Could you check a few things on this model? Use its own coordinates, in mm. A direction names the side the tool comes from. Give positions to 0.01 mm unless a question says otherwise; leave off trailing zeros. Order: outer loops, then holes, each group sorted by start corner. A loop starts at its lowest first (then second) coordinate and runs counter-clockwise, first axis right, second up. Notation, with made-up numbers: (-24, -34.5) -> (17, -34.5) arc R23 cw to (17, -23.5) -> close; hole circle Ø9 at (87, 12). An arc over 180 degrees is marked (long way). Answer as CSV lines item,"result". Start each with the question number.
(1) Will these pins go through, and if not, where does the flat tip stop? pin 1 Ø3 at (x, z) = (7, 27) entering from +Y; pin 2 Ø8.5 at (x, y) = (1.5, 32.5) entering from +Z; pin 3 Ø6.5 at (x, y) = (0, 38) entering from +Z; pin 4 Ø8 at (x, z) = (-3.5, 29.5) entering from -Y.
(2) I want a section at D-D (z = 25.5). Please give me the cut outline in (x, y), plus the area to 3 significant figures.
(3) On a 3-axis mill with a long thin cutter (end or side, diameter ignored), from which of +Z, -Z, +X, -X, +Y, -Y can I reach the whole of each face in a straight line? I mean faces 4 (the face through (-1.2, 0.3, 13.4)), 5 (the face through (0, 2, 26)). Say none if no direction works.
(4) I want a section at C-C (x = -4.5). Please give me the cut outline in (y, z).
(5) I need wall thicknesses on L1, parallel to X at y = 0.35, z = 38; L2, parallel to Y at x = -2, z = 3.5. Which ranges of each line are inside material? Lowest first, please.
(6) We'd pull the mould along Y, two halves only. Please class faces 1 (the face through (-5.94, 0.99, 47.58)), 2 (the face through (-0.12, 0.86, 0.9)), 3 (the face through (-0.434, 36.048, 0.254)): released by +Y, released by -Y, zero draft, split by the parting line, or undercut.
(7) I want a section at A-A (y = 38). Please give me the cut outline in (x, z).
```python
from build123d import *

# Parameters (mm, degrees)
EXTRUDE_1_DEPTH      = 8.5
EXTRUDE_1_DEPTH_BACK = 8.5
SKETCH_3_R           = 2
CUT_EXTRUDE_2_DEPTH  = 15.5
SKETCH_4_R           = 2
CUT_EXTRUDE_3_DEPTH  = 15.5
FILLET_1_R           = 8.5
CHAMFER_1_SIZE       = 1.5


with BuildPart() as part:
    # 草图1 → 凸台-拉伸1 (new, two sides: drawn at the far end of the back side and taken through both)
    with BuildSketch(Plane(origin=(0, 0, 0), x_dir=(0, 0, -1), z_dir=(1, 0, 0)).offset(-EXTRUDE_1_DEPTH_BACK)):
        with BuildLine():
            Line((-50, 0), (-3, 0))
            ThreePointArc((-3, 0), (-0.878679656, 0.878679656), (0, 3))
            Line((0, 3), (0, 50))
            Line((0, 50), (-2, 50))
            Line((-2, 50), (-2, 3))
            ThreePointArc((-2, 3), (-2.292893219, 2.292893219), (-3, 2))
            Line((-3, 2), (-50, 2))
            Line((-50, 2), (-50, 0))
        make_face()
    extrude(amount=EXTRUDE_1_DEPTH + EXTRUDE_1_DEPTH_BACK)

    # 草图3 → 切除-拉伸2 (cut)
    with BuildSketch(Plane(origin=(0, 2, 0), x_dir=(1, 0, 0), z_dir=(0, 1, 0))):
        with Locations(Location((0, -38, 0), (0, 0, 270))):
            Circle(SKETCH_3_R)
        with Locations(Location((0, -15, 0), (0, 0, 270))):
            Circle(SKETCH_3_R)
    extrude(amount=-CUT_EXTRUDE_2_DEPTH, mode=Mode.SUBTRACT)

    # 草图4 → 切除-拉伸3 (cut)
    with BuildSketch(Plane.XY.offset(2)):
        with Locations((0, 38)):
            Circle(SKETCH_4_R)
        with Locations((0, 15)):
            Circle(SKETCH_4_R)
    extrude(amount=-CUT_EXTRUDE_3_DEPTH, mode=Mode.SUBTRACT)

    # 圆角1
    fillet_1_edges = [part.edges().sort_by_distance(p)[0] for p in [
        (8.5, 50, 1),
        (-8.5, 50, 1),
        (8.5, 1, 50),
        (-8.5, 1, 50),
    ]]
    fillet(fillet_1_edges, radius=FILLET_1_R - 0.0001)  # a hair under: the kernel refuses the full size

    # 倒角1
    chamfer_1_edges = [part.edges().sort_by_distance(p)[0] for p in [
        (0, 2, 36),
        (0, 2, 13),
        (-2, 38, 2),
        (-2, 15, 2),
    ]]
    chamfer(chamfer_1_edges, length=CHAMFER_1_SIZE)


solid = part.part
```
Final values:
1,pin 1,"y = 2"
1,pin 2,"z = 2"
1,pin 3,"z = 1.75"
1,pin 4,"y = 0"
2,outline,"(-8.5, 0) -> (8.5, 0) -> (8.5, 2) -> (-8.5, 2) -> close"
2,area,"34.0 mm²"
3,face 4,"+Y, -Y"
3,face 5,"+Z, +X, -X, +Y"
4,outline,"(0, 3) arc R3 ccw to (3, 0) -> (48.71, 0) -> (48.71, 2) -> (3, 2) arc R1 cw to (2, 3) -> (2, 48.71) -> (0, 48.71) -> close"
5,L1,"-8.5 to -2, 2 to 8.5"
5,L2,"0 to 2"
6,face 1,"zero draft"
6,face 2,"released by -Y"
6,face 3,"undercut"
7,outline,"(-8.5, 0) -> (-2, 0) -> (-2, 0.5) -> (-3.5, 2) -> (-8.5, 2) -> close; (2, 0) -> (8.5, 0) -> (8.5, 2) -> (3.5, 2) -> (2, 0.5) -> close"
